The model under review builds one solid part; all positions refer to its coordinate system, in mm. A direction names the side the tool comes from. Give positions to 0.01 mm unless a question says otherwise; leave off trailing zeros. Loops run counter-clockwise (first coordinate to the right, second up) from the corner with the lowest first, then second, coordinate; pieces in that order, holes last. Notation, with made-up numbers: M 9,9.5 L 65,9.5 A18 ccw 65,39.5 Z; hole C -18,69 d11. An arc over 180 degrees is marked long. Put each result on its own line as item: value. Start each with the question number.
```python
from build123d import *

# Parameters (mm, degrees)
EXTRUSION1_DEPTH = 220
ESQUISSE2_R      = 1.5
EXTRUSION2_DEPTH = 200


with BuildPart() as part:
    # Esquisse1 → Extrusion1 (new body)
    with BuildSketch(Plane.XY):
        Polygon((-25.845256994, 11.357120085), (-25.845256994, -8.642879915), (-5.845256994, -8.642879915), (-5.845256994, 11.357120085), (-7.345256994, 11.357120085), (-7.345256994, -7.142879915), (-24.345256994, -7.142879915), (-24.345256994, 11.357120085), align=None)
    extrude(amount=EXTRUSION1_DEPTH)

    # Esquisse2 → Extrusion2 (cut)
    with BuildSketch(Plane.XZ.offset(8.642879915)):
        with Locations(Location((-15.845256994, 210, 0), (0, 0, 270))):
            Circle(ESQUISSE2_R)
        with Locations(Location((-15.845256994, 10, 0), (0, 0, 270))):
            Circle(ESQUISSE2_R)
        with Locations(Location((-15.845256994, 160, 0), (0, 0, 270))):
            Circle(ESQUISSE2_R)
        with Locations(Location((-15.845256994, 110, 0), (0, 0, 270))):
            Circle(ESQUISSE2_R)
        with Locations(Location((-15.845256994, 60, 0), (0, 0, 270))):
            Circle(ESQUISSE2_R)
    extrude(amount=-EXTRUSION2_DEPTH, mode=Mode.SUBTRACT)


solid = part.part
```
Item 1: Draft analysis for pull direction X (two halves, no side actions). For faces 3 (the flat face through (-25.845, 1, 108)), 4 (the flat face through (-7.345, 2, 108)), 5 (the flat face through (-15.9, -7.5, 220)), 6 (the flat face through (-16, -7.143, 108)), state which applies: +X half, -X half, draft (parallel to the pull), parting line (faces both ways), or undercut.
Item 2: Tool access review of faces 1 (the flat face through (-24.345, 2, 108)), 2 (the flat face through (-5.845, 1, 108)): name each direction out of +Z, -Z, +X, -X, +Y, -Y from which nothing blocks a thin tool from reaching the whole face with its end or side.
Item 3: Consider section C-C, the plane x = -20.75. Write out the cut boundary in (y, z).
Item 4: Consider section A-A, the plane y = 1.5. Write out the cut boundary in (x, z).
Item 5: To check wall thickness, follow L1, parallel to X at y = -7.65, z = 160; L2, parallel to X at y = 3, z = 171.5; L3, parallel to Y at x = -23, z = 82. State the ranges of each line that lie inside material, in increasing order. Write a range as [from, to].
Item 6: Clearance check with flat-ended pins moving along their axes: pin 1 Ø2.5 at (x, z) = (-15.85, 160) entering from -Y (1 decimal); pin 2 Ø4 at (x, z) = (-15.85, 10) entering from +Y; pin 3 Ø5 at (x, z) = (-15.85, 210) entering from -Y. State where each tip first meets the part, or that it passes through.
Item 7: Consider section B-B, the plane z = 196. Write out the cut boundary in (x, y).
Report:
1. face 3: -X half
1. face 4: undercut
1. face 5: draft
1. face 6: undercut
2. face 1: +Z, -Z, +Y
2. face 2: +Z, -Z, +X, +Y, -Y
3. outline: M -8.64,0 L -7.14,0 L -7.14,220 L -8.64,220 Z
4. outline: M -25.85,0 L -24.35,0 L -24.35,220 L -25.85,220 Z; M -7.35,0 L -5.85,0 L -5.85,220 L -7.35,220 Z
5. L1: [-25.85, -17.35], [-14.35, -5.85]
5. L2: [-25.85, -24.35], [-7.35, -5.85]
5. L3: [-8.64, -7.14]
6. pin 1: through
6. pin 2: y = -7.14
6. pin 3: y = -8.64
7. outline: M -25.85,-8.64 L -5.85,-8.64 L -5.85,11.36 L -7.35,11.36 L -7.35,-7.14 L -24.35,-7.14 L -24.35,11.36 L -25.85,11.36 Z
